Verification items for the finished model (mm, model axes). A direction names the side the tool comes from. Coordinates: 2 decimals unless noted, no trailing zeros. Order: outer loops, then holes, each group sorted by start corner. A loop starts at its lowest first (then second) coordinate and runs counter-clockwise, first axis right, second up. Notation, with made-up numbers: (47.5, -38.5) -> (67.5, -38.5) arc R22 ccw to (67.5, -3.5) -> close; hole circle Ø8 at (10.25, 49). An arc over 180 degrees is marked (long way). Answer as CSV lines item,"result".
```python
from build123d import *

# Parameters (mm, degrees)
PAD_DEPTH       = 9
POCKET_DEPTH    = 3
SKETCH002_R     = 1.6
POCKET001_DEPTH = 5


with BuildPart() as pocket001:
    # Sketch → Pad (new body)
    with BuildSketch(Plane.XY):
        with BuildLine():
            ThreePointArc((-1, 6.928203), (-5.291503, 4.582576), (-7, 0))
            Line((-10, 0), (-7, 0))
            ThreePointArc((-6.5, 7.599342), (-9.082951, 4.1833), (-10, 0))
            Line((-6.5, 7.599342), (-6.5, 16))
            Line((-6.5, 16), (-1, 16))
            Line((-1, 16), (-1, 6.928203))
        make_face()
    extrude(amount=PAD_DEPTH)

    # Sketch001 → Pocket (cut)
    with BuildSketch(Plane(origin=(-6.5, 0, 0), x_dir=(0, -1, 0), z_dir=(-1, 0, 0))):
        Polygon((-13.232051, 7.5), (-9.767949, 7.5), (-8.035898, 4.5), (-9.767949, 1.5), (-13.232051, 1.5), (-14.964102, 4.5), align=None)
    extrude(amount=-POCKET_DEPTH, mode=Mode.SUBTRACT)

    # Sketch002 → Pocket001 (cut)
    with BuildSketch(Plane(origin=(-3.5, 0, 0), x_dir=(0, -1, 0), z_dir=(-1, 0, 0))):
        with Locations((-11.5, 4.5)):
            Circle(SKETCH002_R)
    extrude(amount=-POCKET001_DEPTH, mode=Mode.SUBTRACT)


with BuildPart() as part_mirroring:
    # Part__Mirroring: instance of Pocket001
    add(pocket001.part.mirror(Plane(origin=(0, 0, 0), x_dir=(1, 0, 0), z_dir=(0, 1, 0))))


with BuildPart() as fusion:
    # Fusion base: copy of Pocket001
    add(pocket001.part)

    # Fusion: union Part__Mirroring
    add(part_mirroring.part)


solid = fusion.part
```
Item 1: Section check C-C, the plane z = 3.5. Record the boundary of the cut face in (x, y), plus the area to 3 significant figures.
Answer list:
outline,"(-7, 0) arc R7 cw to (-1, 6.93) -> (-1, 10.25) -> (-3.5, 10.25) -> (-3.5, 8.61) -> (-6.5, 8.61) -> (-6.5, 7.6) arc R10 ccw to (-6.5, -7.6) -> (-6.5, -8.61) -> (-3.5, -8.61) -> (-3.5, -10.25) -> (-1, -10.25) -> (-1, -6.93) arc R7 cw to start; (-6.5, -16) -> (-1, -16) -> (-1, -12.75) -> (-3.5, -12.75) -> (-3.5, -14.39) -> (-6.5, -14.39) -> close; (-6.5, 14.39) -> (-3.5, 14.39) -> (-3.5, 12.75) -> (-1, 12.75) -> (-1, 16) -> (-6.5, 16) -> close"
area,"103 mm2"
Item 2: Tool access check on faces 1 (the flat face through (-5, -12, 7.5)), 2 (the flat face through (-7.4, -0.2, 0)), 3 (the flat face through (-6.5, -15, 3)). Record the directions out of +Z, -Z, +X, -X, +Y, -Y that give a thin tool (end or side, any length) a straight path to the whole face; none if there is none.
Answer list:
face 1,"-X"
face 2,"-Z, +X, -X, +Y, -Y"
face 3,"+Z, -Z, -X, -Y"
Item 3: Section check D-D, the plane y = -14. Record the boundary of the cut face in (x, z), plus the area to 3 significant figures.
Answer list:
outline,"(-6.5, 0) -> (-1, 0) -> (-1, 9) -> (-6.5, 9) -> (-6.5, 6.17) -> (-3.5, 6.17) -> (-3.5, 2.83) -> (-6.5, 2.83) -> close"
area,"39.5 mm2"
Item 4: Release check for a two-part mould opening along Y. For faces 4 (the flat face through (-5, -14.1, 6)), 5 (the cylindrical face through (-2.27, -13.1, 4.57)), 6 (the flat face through (-1, 11.5, 6.4)), 7 (the flat face through (-4, 16, 4)) record: +Y half, -Y half, draft (parallel to the pull), parting line (faces both ways), or undercut.
Answer list:
face 4,"undercut"
face 5,"undercut"
face 6,"draft"
face 7,"+Y half"
Item 5: Thickness scan on line 1 (Z direction, x = -2.35, y = -11.5); line 2 (Y direction, x = -3.25, z = 5.5); line 3 (Y direction, x = -5, z = 5.25). Record the ranges inside material, lowest first.
Answer list:
line 1,"0 to 2.9, 6.1 to 9"
line 2,"-16 to -12.75, -10.25 to -6.2, 6.2 to 10.25, 12.75 to 16"
line 3,"-16 to -14.53, -8.47 to -4.9, 4.9 to 8.47, 14.53 to 16"
Item 6: Depth check by flat-ended pin: pin 1 Ø3 at (y, z) = (-11.5, 4.5) entering from -X; pin 2 Ø4 at (y, z) = (-8.5, 5.5) entering from -X; pin 3 Ø3.5 at (x, y) = (-4.5, 11) entering from -Z; pin 4 Ø2 at (y, z) = (4, 6) entering from -X. Enter the tip coordinate at first touch or a pass-through.
Answer list:
pin 1,"through"
pin 2,"x = -7.6"
pin 3,"z = 0"
pin 4,"x = -9.54"
Item 7: Section check B-B, the plane x = -2.5. Record the boundary of the cut face in (y, z), plus the area to 3 significant figures.
Answer list:
outline,"(-16, 0) -> (-6.54, 0) -> (-6.54, 9) -> (-16, 9) -> close; (6.54, 0) -> (16, 0) -> (16, 9) -> (6.54, 9) -> close; hole circle Ø3.2 at (-11.5, 4.5); hole circle Ø3.2 at (11.5, 4.5)"
area,"154 mm2"
Item 8: Section check A-A, the plane y = 11.5. Record the boundary of the cut face in (x, z).
Answer list:
outline,"(-6.5, 0) -> (-1, 0) -> (-1, 2.9) -> (-3.5, 2.9) -> (-3.5, 1.5) -> (-6.5, 1.5) -> close; (-6.5, 7.5) -> (-3.5, 7.5) -> (-3.5, 6.1) -> (-1, 6.1) -> (-1, 9) -> (-6.5, 9) -> close"
